Can you work these out from the drawing? Everything is in mm from the part's minimum corner. A direction names the side the tool comes from. Give positions to 0.01 mm unless a question says otherwise; leave off trailing zeros. Write each loop counter-clockwise with the first axis right and the second up, starting at its lowest first coordinate (ties: lowest second). Pieces come first, ordered by that corner, then holes. Notation, with made-up numbers: (20.25, 37) - (39.25, 37) arc R25 cw to (39.25, 66) - close; hole circle Ø1 at (-36.5, 19). An arc over 180 degrees is marked (long way). Answer in a Markdown table with one row per item.
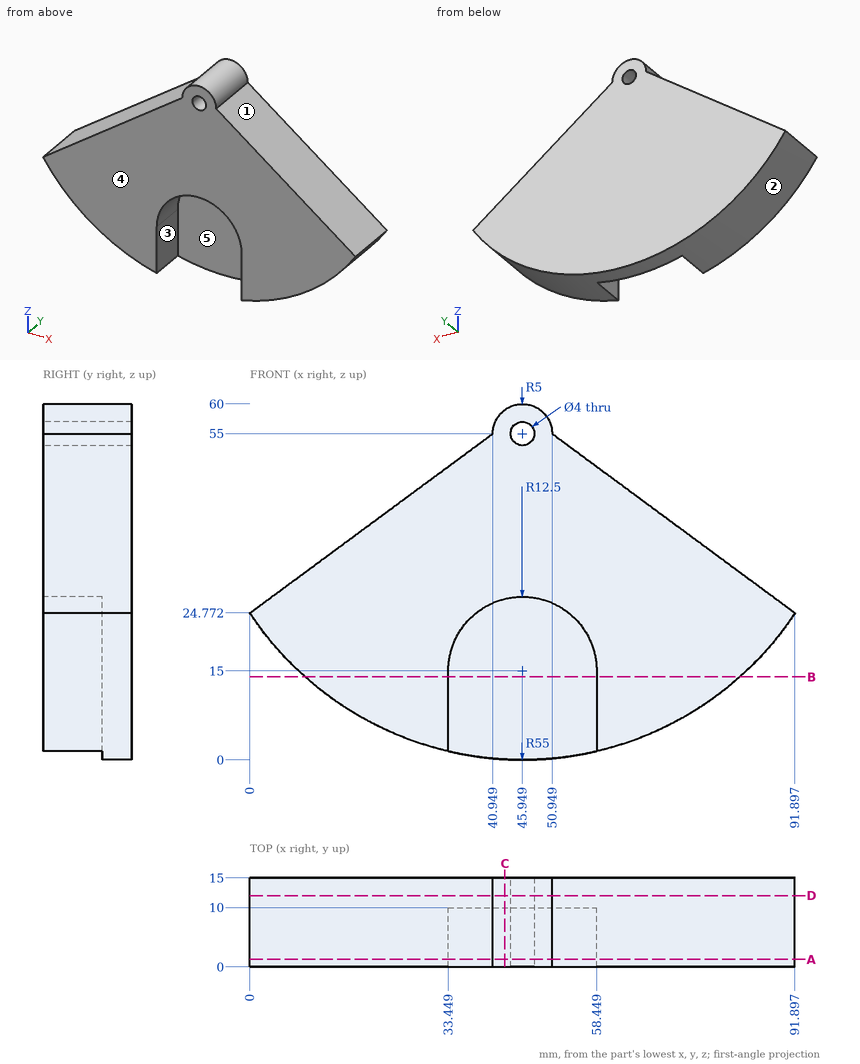
1) We'd pull the mould along X, two halves only. Please class the marked faces 1, 2 and 3: +X half, -X half, draft (parallel to the pull), parting line (faces both ways), or undercut.
Check values:
| item | result |
|---|---|
| face 1 | +X half |
| face 2 | parting line |
| face 3 | undercut |
2) Imagine slicing it at A-A (y = 1.25). List the corners of the cut face in (x, z) for me.
Check values:
| item | result |
|---|---|
| outline | (0, 24.77) arc R55 ccw to (33.45, 1.44) - (33.45, 15) arc R12.5 cw to (58.45, 15) - (58.45, 1.44) arc R55 ccw to (91.9, 24.77) - (50.95, 55) arc R5 ccw to (40.95, 55) - close; hole circle Ø4 at (45.95, 55) |
3) On a 3-axis mill with a long thin cutter (end or side, diameter ignored), from which of +Z, -Z, +X, -X, +Y, -Y can I reach the whole of each face in a straight line? I mean the marked faces 4 and 5. Say none if no direction works.
Check values:
| item | result |
|---|---|
| face 4 | +Z, -Z, +X, -X, -Y |
| face 5 | -Z, -Y |
4) If I drill on line 1 (X direction, y = 4, z = 20) (1 decimal); line 2 (Z direction, x = 9, y = 3.75) (1 decimal); line 3 (Y direction, x = 49, z = 7.5), over which ranges is the centre line in solid material (lowest first)?
Check values:
| item | result |
|---|---|
| line 1 | x = 3.5 to 34.5, 57.4 to 88.4 |
| line 2 | z = 14.3 to 31.4 |
| line 3 | y = 10 to 15 |
5) Imagine slicing it at C-C (x = 43). List the corners of the cut face in (y, z) for me, then the cut area to 3 significant figures.
Check values:
| item | result |
|---|---|
| outline | (0, 27.15) - (10, 27.15) - (10, 0.08) - (15, 0.08) - (15, 59.04) - (0, 59.04) - close |
| area | 614 mm2 |
6) Imagine slicing it at B-B (z = 14). List the corners of the cut face in (x, y) for me, then the cut area to 3 significant figures.
Check values:
| item | result |
|---|---|
| outline | (9.29, 0) - (33.45, 0) - (33.45, 10) - (58.45, 10) - (58.45, 0) - (82.61, 0) - (82.61, 15) - (9.29, 15) - close |
| area | 850 mm2 |
7) Imagine slicing it at D-D (y = 12). List the corners of the cut face in (x, z) for me.
Check values:
| item | result |
|---|---|
| outline | (0, 24.77) arc R55 ccw to (91.9, 24.77) - (50.95, 55) arc R5 ccw to (40.95, 55) - close; hole circle Ø4 at (45.95, 55) |
8) Will these pins go through, and if not, where does the flat tip stop? P1, Ø2.5, axis at x = 45.95, z = 55, coming from the -Y side; P2, Ø3, axis at x = 82, y = 9.5, coming from the -Z side; P3, Ø1.5, axis at y = 3, z = 51, coming from the +X side (1 decimal); P4, Ø8, axis at y = 6.5, z = 8.5, coming from the +X side.
Check values:
| item | result |
|---|---|
| P1 | passes through |
| P2 | stops at z = 12.21 |
| P3 | stops at x = 57.4 |
| P4 | stops at x = 80.86 |
